Can you work these out from the model? Positions are in its coordinate system, mm. Give positions to 0.01 mm unless a question says otherwise; leave off trailing zeros. Loops run counter-clockwise (first coordinate to the right, second up) from the corner with the lowest first, then second, coordinate; pieces in that order, holes last.
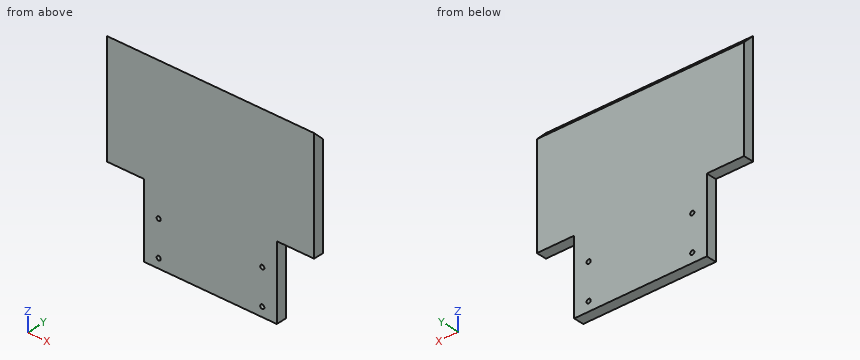
from build123d import *

# Parameters (mm, degrees)
CROQUIS2_W              = 100
CROQUIS2_H              = 99.2
SALIENTE_EXTRUIR1_DEPTH = 5
CHAFL_N1_SIZE           = 5
CROQUIS3_W              = 18
CROQUIS3_H              = 45.2
CORTAR_EXTRUIR1_DEPTH   = 5
CROQUIS6_R              = 1
CORTAR_EXTRUIR3_DEPTH   = 10
CROQUIS8_W              = 64
CROQUIS8_H              = 9.6
CORTAR_EXTRUIR4_DEPTH   = 141.94552139


with BuildPart() as part:
    # Croquis2 → Saliente-Extruir1 (new body)
    with BuildSketch(Plane(origin=(0, 0, 0), x_dir=(1, 0, 0), z_dir=(0, 1, 0))):
        with Locations((50, 49.6)):
            Rectangle(CROQUIS2_W, CROQUIS2_H)
    extrude(amount=SALIENTE_EXTRUIR1_DEPTH)

    # Chaflán1
    chafl_n1_edges = [part.edges().sort_by_distance(p)[0] for p in [
        (50, 5, 0),
    ]]
    chamfer(chafl_n1_edges, length=CHAFL_N1_SIZE - 0.0001)  # a hair under: the kernel refuses the full size

    # Croquis3 → Cortar-Extruir1 (cut)
    with BuildSketch(Plane(origin=(0, 5, 0), x_dir=(1, 0, 0), z_dir=(0, 1, 0))):
        with Locations((9, 76.6)):
            Rectangle(CROQUIS3_W, CROQUIS3_H)
        with Locations((91, 76.6)):
            Rectangle(CROQUIS3_W, CROQUIS3_H)
    extrude(amount=-CORTAR_EXTRUIR1_DEPTH, mode=Mode.SUBTRACT)

    # Croquis6 → Cortar-Extruir3 (cut)
    with BuildSketch(Plane(origin=(0, 5, 0), x_dir=(1, 0, 0), z_dir=(0, 1, 0))):
        with Locations(Location((25, 85.1, 0), (0, 0, 270))):
            Circle(CROQUIS6_R)
        with Locations(Location((25, 68.1, 0), (0, 0, 270))):
            Circle(CROQUIS6_R)
        with Locations(Location((75, 85.1, 0), (0, 0, 270))):
            Circle(CROQUIS6_R)
        with Locations(Location((75, 68.1, 0), (0, 0, 270))):
            Circle(CROQUIS6_R)
    extrude(amount=-CORTAR_EXTRUIR3_DEPTH, mode=Mode.SUBTRACT)

    # Croquis8 → Cortar-Extruir4 (cut, through all)
    with BuildSketch(Plane(origin=(0, 5, 0), x_dir=(1, 0, 0), z_dir=(0, 1, 0))):
        with Locations((50, 94.4)):
            Rectangle(CROQUIS8_W, CROQUIS8_H)
    extrude(amount=-CORTAR_EXTRUIR4_DEPTH, mode=Mode.SUBTRACT)


solid = part.part
(1) Suppose I cut it at A-A on y = 2.95. List the corners of the cut face in (x, z) for me.
Returned:
outline: (0, -54) - (18, -54) - (18, -89.6) - (82, -89.6) - (82, -54) - (100, -54) - (100, -2.95) - (0, -2.95) - close; hole circle Ø2 at (25, -85.1); hole circle Ø2 at (25, -68.1); hole circle Ø2 at (75, -85.1); hole circle Ø2 at (75, -68.1)
(2) Please list where these lines run through material, in increasing order: probe 1 along X at (y, z) = (2.35, -68.1); probe 2 along Z at (x, y) = (75, 2.75); probe 3 along Z at (x, y) = (75, 3.4).
Returned:
probe 1: x = 18 to 24, 26 to 74, 76 to 82
probe 2: z = -89.6 to -86.1, -84.1 to -69.1, -67.1 to -2.75
probe 3: z = -89.6 to -86.1, -84.1 to -69.1, -67.1 to -3.4
(3) Will these pins go through, and if not, where does the flat tip stop? P1, Ø1, axis at x = 86.5, y = 2.5, coming from the +Z side; P2, Ø1.6, axis at x = 25, z = -68.1, coming from the -Y side; P3, Ø1.5, axis at x = 26, y = 2, coming from the +Z side; P4, Ø2.5, axis at x = 92, y = 2, coming from the -Z side.
Returned:
P1: stops at z = -2
P2: passes through
P3: stops at z = -1.25
P4: stops at z = -54
(4) Suppose I cut it at C-C on z = -72.5. List the corners of the cut face in (x, y) for me, plus the area to 3 significant figures.
Returned:
outline: (18, 0) - (82, 0) - (82, 5) - (18, 5) - close
area: 320 mm2
